Build history of the part. All positions in model axes, mm. A direction names the side the tool comes from. Round coordinates to 2 decimals unless told otherwise and drop trailing zeros. Write each loop counter-clockwise with the first axis right and the second up, starting at its lowest first coordinate (ties: lowest second). Pieces come first, ordered by that corner, then holes.
Item 1: Band-saw the part on C-C, the plane y = 0.5. Write the cut outline in (x, z).
Item 2: Mould opens along Y. For faces 4 (the flat face through (-203, 25.4, -12)), 5 (the flat face through (-24, 63.5, 0.2)), 6 (the flat face through (-198.438, -44, -13)), 7 (the flat face through (-203, -25.4, -12)) say: +Y half, -Y half, draft (parallel to the pull), parting line (faces both ways), or undercut.
Item 3: 3-axis set-ups, long thin cutter, end or side, ignore diameter. For faces 1 (the cylindrical face through (-203.3, 44.72, -30.16)), 2 (the flat face through (-207.962, -44, -13)), 3 (the flat face through (-198.438, 45, -13)): which of +Z, -Z, +X, -X, +Y, -Y reach the whole face in a straight line?
Item 4: Wall check: probe 1 along X at (y, z) = (-43.5, -25.4) (1 decimal); probe 2 along X at (y, z) = (-32, -25); probe 3 along Z at (x, y) = (-203, -51). Give the ranges that are in metal, low to high.
Item 5: Drop flat-ended pins along their axis: pin 1 Ø10 at (x, y) = (140, -26.5) entering from -Z; pin 2 Ø7.5 at (y, z) = (48.5, -9) entering from -X; pin 3 Ø10 at (y, z) = (-39, -5.5) entering from +X; pin 4 Ø10 at (x, z) = (-177.5, -8.5) entering from -Y. Give the stop position or say it passes through.
Item 6: Band-saw the part on B-B, the plane x = -242. Write the cut outline in (y, z), then the cut area to 3 significant figures.
```python
from build123d import *

# Parameters (mm, degrees)
SKETCH1_W           = 609.6
SKETCH1_H           = 127
BOSS_EXTRUDE2_DEPTH = 4.7625
SKETCH3_R           = 3.175
BOSS_EXTRUDE3_DEPTH = 63.5
SKETCH4_W           = 30.1625
SKETCH4_H           = 50.8
CUT_EXTRUDE1_DEPTH  = 107.3625


with BuildPart() as part:
    # Sketch1 → Boss-Extrude2 (new body)
    with BuildSketch(Plane.XY):
        Rectangle(SKETCH1_W, SKETCH1_H)
    extrude(amount=BOSS_EXTRUDE2_DEPTH)

    # Sketch3 → Boss-Extrude3 (add, symmetric)
    with BuildSketch(Plane(origin=(0, 0, 0), x_dir=(1, 0, 0), z_dir=(0, 1, 0))):
        with BuildLine():
            Line((-207.9625, 0), (-207.9625, 25.4))
            ThreePointArc((-207.9625, 25.4), (-203.2, 30.1625), (-198.4375, 25.4))
            Line((-198.4375, 25.4), (-198.4375, 0))
            Line((-198.4375, 0), (-207.9625, 0))
        make_face()
        with Locations((-203.2, 25.4)):
            Circle(SKETCH3_R, mode=Mode.SUBTRACT)
    extrude(amount=BOSS_EXTRUDE3_DEPTH, both=True)

    # Sketch4 → Cut-Extrude1 (cut, through all)
    with BuildSketch(Plane(origin=(-198.4375, 0, 0), x_dir=(0, 0, -1), z_dir=(1, 0, 0))):
        with Locations((15.08125, 0)):
            Rectangle(SKETCH4_W, SKETCH4_H)
    extrude(amount=-CUT_EXTRUDE1_DEPTH, mode=Mode.SUBTRACT)


solid = part.part
```
Results:
1. outline: (-304.8, 0) - (304.8, 0) - (304.8, 4.76) - (-304.8, 4.76) - close
2. face 4: undercut
2. face 5: +Y half
2. face 6: draft
2. face 7: undercut
3. face 1: -Z, +Y, -Y
3. face 2: -Z, -X, +Y, -Y
3. face 3: -Z, +X, +Y, -Y
4. probe 1: x = -208 to -206.4, -200 to -198.4
4. probe 2: x = -207.96 to -206.35, -200.05 to -198.44
4. probe 3: z = -30.16 to -28.57, -22.23 to 4.76
5. pin 1: stops at z = 0
5. pin 2: stops at x = -207.96
5. pin 3: stops at x = -198.44
5. pin 4: passes through
6. outline: (-63.5, 0) - (63.5, 0) - (63.5, 4.76) - (-63.5, 4.76) - close
6. area: 605 mm2
